```python
from build123d import *

# Parameters (mm, degrees)
SKETCH1_W           = 80
SKETCH1_H           = 80
BOSS_EXTRUDE1_DEPTH = 1.6
SKETCH2_R           = 10
SKETCH2_R_2         = 6
BOSS_EXTRUDE2_DEPTH = 12
SKETCH3_W           = 23.33
SKETCH3_H           = 20
SKETCH3_W_2         = 23.34
SKETCH3_W_3         = 17.33
CUT_EXTRUDE1_DEPTH  = 12
BOSS_EXTRUDE3_DEPTH = 12
SKETCH5_W           = 6
SKETCH5_H           = 1.4
BOSS_EXTRUDE4_DEPTH = 12
SKETCH6_W           = 16
SKETCH6_H           = 14
BOSS_EXTRUDE5_DEPTH = 2
CHAMFER1_SIZE       = 2
SKETCH7_W           = 4
SKETCH7_H           = 1.4
BOSS_EXTRUDE6_DEPTH = 3.5
CHAMFER2_SIZE       = 5
BOSS_EXTRUDE7_DEPTH = 3


with BuildPart() as part:
    # Sketch1 → Boss-Extrude1 (new body)
    with BuildSketch(Plane.XY):
        Rectangle(SKETCH1_W, SKETCH1_H)
    extrude(amount=BOSS_EXTRUDE1_DEPTH)

    # Sketch2 → Boss-Extrude2 (add)
    with BuildSketch(Plane.XY.offset(1.6)):
        Circle(SKETCH2_R)
        Circle(SKETCH2_R_2, mode=Mode.SUBTRACT)
    extrude(amount=BOSS_EXTRUDE2_DEPTH)

    # Sketch3 → Cut-Extrude1 (cut)
    with BuildSketch(Plane.XY.offset(1.6)):
        with Locations((-23.335, 26)):
            Rectangle(SKETCH3_W, SKETCH3_H)
        with Locations((23.33, 26)):
            Rectangle(SKETCH3_W_2, SKETCH3_H)
        with Locations((-0.005, 26)):
            Rectangle(SKETCH3_W_3, SKETCH3_H)
    extrude(amount=-CUT_EXTRUDE1_DEPTH, mode=Mode.SUBTRACT)

    # Sketch4 → Boss-Extrude3 (add)
    with BuildSketch(Plane.XY.offset(1.6)):
        Polygon((-5, -40), (-5, -25), (-5, -22), (-8, -22), (-8, -40), align=None)
        Polygon((5, -40), (5, -25), (5, -22), (8, -22), (8, -40), align=None)
    extrude(amount=BOSS_EXTRUDE3_DEPTH)

    # Sketch5 → Boss-Extrude4 (add)
    with BuildSketch(Plane.XY.offset(1.6)):
        with Locations((-5, -21.3)):
            Rectangle(SKETCH5_W, SKETCH5_H)
        with Locations((5, -21.3)):
            Rectangle(SKETCH5_W, SKETCH5_H)
    extrude(amount=BOSS_EXTRUDE4_DEPTH)

    # Sketch6 → Boss-Extrude5 (add)
    with BuildSketch(Plane.XY.offset(13.6)):
        with Locations((0, -27.6)):
            Rectangle(SKETCH6_W, SKETCH6_H)
    extrude(amount=BOSS_EXTRUDE5_DEPTH)

    # Chamfer1
    chamfer1_edges = [part.edges().sort_by_distance(p)[0] for p in [
        (6.5, -34.6, 13.6),
        (-6.5, -34.6, 13.6),
    ]]
    chamfer(chamfer1_edges, length=CHAMFER1_SIZE - 0.0001)  # a hair under: the kernel refuses the full size

    # Sketch7 → Boss-Extrude6 (add)
    with BuildSketch(Plane(origin=(0, 0, 13.6), x_dir=(-1, 0, 0), z_dir=(0, 0, -1))):
        with Locations((0, -21.3)):
            Rectangle(SKETCH7_W, SKETCH7_H)
    extrude(amount=BOSS_EXTRUDE6_DEPTH)

    # Chamfer2
    chamfer2_edges = [part.edges().sort_by_distance(p)[0] for p in [
        (8, -30.3, 1.6),
        (-8, -30.3, 1.6),
    ]]
    chamfer(chamfer2_edges, length=CHAMFER2_SIZE)

    # Sketch8 → Boss-Extrude7 (add)
    with BuildSketch(Plane.XY.offset(1.6)):
        Polygon((-13, -36.339774094), (-13, -40), (-40, -40), (-40, 40), (40, 40), (40, -40), (13, -40), (13, -36.339774094), (38, -36.339774094), (38, 38), (-38, 38), (-38, -36.339774094), align=None)
    extrude(amount=BOSS_EXTRUDE7_DEPTH)


solid = part.part
```
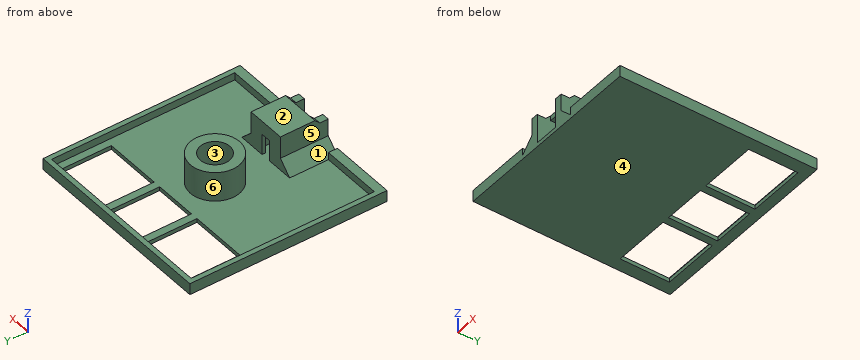
Verification items for the finished model (mm, model axes). Face numbers are marked on the shaded views. A direction names the side the tool comes from. Give positions to 0.01 mm unless a question says otherwise; leave off trailing zeros. Order: outer loops, then holes, each group sorted by start corner. A loop starts at its lowest first (then second) coordinate and runs counter-clockwise, first axis right, second up. Notation, with made-up numbers: (12, 88.25) -> (20, 88.25) arc R16 cw to (20, 99.25) -> close; hole circle Ø7 at (9, 76.5). An arc over 180 degrees is marked (long way). Use a Markdown table: item, result.
1) Section check B-B, the plane z = 3. Record the boundary of the cut face in (x, y), then the cut area to 3 significant figures.
Results:
| item | result |
|---|---|
| outline | (-40, -40) -> (-13, -40) -> (-13, -36.34) -> (-38, -36.34) -> (-38, 38) -> (38, 38) -> (38, -36.34) -> (13, -36.34) -> (13, -40) -> (40, -40) -> (40, 40) -> (-40, 40) -> close; (-11.6, -40) -> (-5, -40) -> (-5, -22) -> (-2, -22) -> (-2, -20.6) -> (-11.6, -20.6) -> close; circle Ø20 at (0, 0); (2, -22) -> (5, -22) -> (5, -40) -> (11.6, -40) -> (11.6, -20.6) -> (2, -20.6) -> close; hole circle Ø12 at (0, 0) |
| area | 1,120 mm² |
2) Section check C-C, the plane y = 31. Record the boundary of the cut face in (x, z).
Results:
| item | result |
|---|---|
| outline | (-40, 0) -> (-35, 0) -> (-35, 1.6) -> (-38, 1.6) -> (-38, 4.6) -> (-40, 4.6) -> close; (-11.67, 0) -> (-8.67, 0) -> (-8.67, 1.6) -> (-11.67, 1.6) -> close; (8.66, 0) -> (11.66, 0) -> (11.66, 1.6) -> (8.66, 1.6) -> close; (35, 0) -> (40, 0) -> (40, 4.6) -> (38, 4.6) -> (38, 1.6) -> (35, 1.6) -> close |
3) Depth check by flat-ended pin: pin 1 Ø24 at (x, y) = (-0.5, 8.5) entering from +Z; pin 2 Ø6 at (x, z) = (15.5, 12.5) entering from -Y (3 decimals); pin 3 Ø2 at (x, y) = (26.5, -8) entering from +Z; pin 4 Ø5 at (y, z) = (11.5, 10.5) entering from -X. Enter the tip coordinate at first touch or a pass-through.
Results:
| item | result |
|---|---|
| pin 1 | z = 13.6 |
| pin 2 | through |
| pin 3 | z = 1.6 |
| pin 4 | x = -4.36 |
4) Section check D-D, the plane z = 12.25. Record the boundary of the cut face in (x, y).
Results:
| item | result |
|---|---|
| outline | circle Ø20 at (0, 0); (-8, -40) -> (-5, -40) -> (-5, -22) -> (5, -22) -> (5, -40) -> (8, -40) -> (8, -20.6) -> (-8, -20.6) -> close; hole circle Ø12 at (0, 0) |
5) Section check A-A, the plane x = 32. Record the boundary of the cut face in (y, z).
Results:
| item | result |
|---|---|
| outline | (-40, 0) -> (16, 0) -> (16, 1.6) -> (-36.34, 1.6) -> (-36.34, 4.6) -> (-40, 4.6) -> close; (36, 0) -> (40, 0) -> (40, 4.6) -> (38, 4.6) -> (38, 1.6) -> (36, 1.6) -> close |
6) Tool access check on the marked faces 1, 2 and 3. Record the directions out of +Z, -Z, +X, -X, +Y, -Y that give a thin tool (end or side, any length) a straight path to the whole face; none if there is none.
Results:
| item | result |
|---|---|
| face 1 | +Z, -Y |
| face 2 | +Z, +X, -X, +Y, -Y |
| face 3 | +Z |
7) Material ranges on probe 1 along X at (y, z) = (31, 2.75); probe 2 along Y at (x, z) = (15, 1.25); probe 3 along Z at (x, y) = (21.5, 3), recorded low to high.
Results:
| item | result |
|---|---|
| probe 1 | -40 to -38, 38 to 40 |
| probe 2 | -40 to 16, 36 to 40 |
| probe 3 | 0 to 1.6 |
8) Mould release check, pull along X, two halves, no side actions. Record for the marked faces 4, 5 and 6: pulls with the +X half, pulls with the -X half, needs draft (parallel to the pull), parting line crosses it, or undercut.
Results:
| item | result |
|---|---|
| face 4 | needs draft |
| face 5 | pulls with the -X half |
| face 6 | undercut |
